Geometry check sheet. Reference: the model listing, model coordinates, mm. A direction names the side the tool comes from. Round coordinates to 2 decimals unless told otherwise and drop trailing zeros. Write each loop counter-clockwise with the first axis right and the second up, starting at its lowest first coordinate (ties: lowest second). Pieces come first, ordered by that corner, then holes. Notation, with made-up numbers: (-40, 88) -> (7, 88) arc R12 ccw to (7, 109) -> close; hole circle Ø10 at (-7.75, 87). An arc over 180 degrees is marked (long way). Return JSON: item names as keys, results as strings. Group by question number.
Autodesk Inventor part; units mm, degrees
ref_plane "YZ Plane" through (0, 0, 0) normal (1, 0, 0) x (0, 1, 0)
ref_plane "XZ Plane" through (0, 0, 0) normal (0, 1, 0) x (-1, 0, 0)
ref_plane "XY Plane" through (0, 0, 0) normal (0, 0, 1) x (1, 0, 0)
sketch "Sketch1" plane through (0, 0, 0) normal (0, 1, 0) x (-1, 0, 0)
  line L0 (-8.3746, 16.5585) -> (42.4254, 16.5585)
  line L1 (42.4254, 16.5585) -> (42.4254, 14.0185)
  line L2 (42.4254, 14.0185) -> (33.5354, 14.0185)
  line L3 (33.5354, 14.0185) -> (33.5354, -11.3815)
  line L4 (33.5354, -11.3815) -> (42.4254, -11.3815)
  line L5 (42.4254, -11.3815) -> (42.4254, -13.9215)
  line L6 (42.4254, -13.9215) -> (-8.3746, -13.9215)
  line L7 (-8.3746, 16.5585) -> (-8.3746, 14.0185)
  line L8 (-8.3746, 14.0185) -> (23.3754, 14.0185)
  line L9 (23.3754, 14.0185) -> (23.3754, -11.3815)
  line L10 (23.3754, -11.3815) -> (-8.3746, -11.3815)
  line L11 (-8.3746, -11.3815) -> (-8.3746, -13.9215)
  point P0 (0, 0)
  dimension "d0" = 30.48
  dimension "d1" = 2.54
  dimension "d2" = 2.54
  dimension "d4" = 2.54
  dimension "d5" = 2.54
  dimension "d6" = 8.89
  dimension "d7" = 50.8
  dimension "d8" = 31.75
extrude "Extrusion1" add sketch "Sketch1" along normal blind 25.4
sketch "Sketch4" plane through (8.3746, 0, -13.9215) normal (0, 0, -1) x (-1, 0, 0)
  line L0 (50.8, 0) -> (0, 0)
  line L1 (50.8, 0) -> (50.8, 25.4)
  line L2 (0, 25.4) -> (50.8, 25.4)
  line L3 (50.8, 25.4) -> (31.75, 25.4)
  line L4 (31.75, 25.4) -> (31.75, 0)
  line L5 (31.75, 0) -> (50.8, 0)
  line L6 (50.8, 0) -> (50.8, 25.4)
  point P0 (8.3746, 0)
  dimension "d56" = 19.05
extrude "Extrusion3" add sketch "Sketch4" along normal blind 13.97
sketch "Sketch5" plane through (-42.4254, 0, 16.5585) normal (0, 0, 1) x (1, 0, 0)
  line L0 (50.8, 0) -> (50.8, 25.4)
  line L1 (50.8, 0) -> (0, 0)
  point P0 (40.64, 12.7)
  dimension "d11" = 10.16
  dimension "d12" = 12.7
hole "Hole1" at (-1.7854, 12.7, 16.5585) direction (0, 0, -1) diameter 9.779 end through all
sketch "Sketch6" plane through (-42.4254, 0, 16.5585) normal (0, 0, 1) x (1, 0, 0)
  line L0 (0, 0) -> (0, 25.4)
  line L1 (50.8, 0) -> (0, 0)
  point P0 (4, 4)
  dimension "d20" = 4
  dimension "d21" = 4
hole "Hole2" at (-38.4254, 4, 16.5585) direction (0, 0, -1) diameter 4.5 end through all
sketch "Sketch2" plane through (-42.4254, 0, 16.5585) normal (0, 0, 1) x (1, 0, 0)
  circle A0 centre (40.64, 12.7) radius 4.8895
  line L0 (40.64, 22.225) -> (40.64, 3.175) construction
  circle A1 centre (40.64, 12.7) radius 4.8895 construction
  line L1 (40.64, 12.7) -> (33.9048, 19.4352) construction
  line L2 (40.64, 12.7) -> (33.9048, 5.9648) construction
  line L3 (40.64, 12.7) -> (47.3752, 5.9648) construction
  line L4 (40.64, 12.7) -> (47.3752, 19.4352) construction
  point P0 (42.4254, 0)
  dimension "d29" = 9.525
  dimension "d30" = 0
  dimension "d33" = 360
  dimension "d60" = 45
  dimension "d63" = 360
hole "Hole3" at (-1.7854, 3.175, 16.5585) at (-1.7854, 22.225, 16.5585) at (-8.5206, 5.9648, 16.5585) at (-8.5206, 19.4352, 16.5585) at (4.9498, 19.4352, 16.5585) at (4.9498, 5.9648, 16.5585) direction (0, 0, -1) diameter 2.794 end through all
fillet "Fillet2" radius 3.175 8 edges at (-42.4254, 0, -19.6365) (-42.4254, 0, 15.2885) (-23.3754, 12.7, 14.0185) (-23.3754, 12.7, -11.3815) (8.3746, 0, -12.6515) (8.3746, 25.4, -12.6515) (8.3746, 25.4, 15.2885) (8.3746, 0, 15.2885)
hole "Hole4" at (-33.5354, 22.1488, 1.9535) direction (1, 0, 0) diameter 3.81 end through all
sketch "Sketch7" plane through (8.3746, 0, -27.8915) normal (0, 0, -1) x (-1, 0, 0)
  circle A0 centre (46.0375, 19.1807) radius 1.45
  circle A1 centre (46.0375, 12.5767) radius 1.524
  line L0 (50.8, 3.175) -> (50.8, 25.4) construction
  line L1 (31.75, 25.4) -> (31.75, 0) construction
  line L2 (50.8, 25.4) -> (31.75, 25.4) construction
  point P0 (8.3746, 0)
  dimension "d65" = 2.9
  dimension "d66" = 3.048
  dimension "d67" = 6.604
  dimension "d69" = 4.7625
  dimension "d71" = 6.2193
extrude "Extrusion4" cut sketch "Sketch7" against normal up to surface (16.51 mm away)
sketch "Sketch9" plane through (8.3746, 0, -27.8915) normal (0, 0, -1) x (-1, 0, 0)
  circle A0 centre (38.1, 12.446) radius 1.45
  line L0 (50.8, 25.4) -> (31.75, 25.4)
  line L1 (50.8, 3.175) -> (50.8, 25.4)
  point P0 (8.3746, 0)
  dimension "d78" = 2.9
  dimension "d79" = 12.954
  dimension "d80" = 12.7
extrude "Extrusion6" cut sketch "Sketch9" against normal blind 12.7
sketch "Sketch10" plane through (0, 25.4, 0) normal (0, 1, 0) x (1, 0, 0)
  line L0 (-42.4254, 11.3815) -> (-42.4254, 27.8915)
  line L1 (-23.3754, 13.9215) -> (-23.3754, 27.8915)
  line L2 (-42.4254, 27.8915) -> (-23.3754, 27.8915)
  line L3 (-23.3754, 27.8915) -> (-23.3754, 26.6215)
  line L4 (-23.3754, 26.6215) -> (-42.4254, 26.6215)
  line L5 (-42.4254, 26.6215) -> (-42.4254, 27.8915)
  point P0 (0, 0)
  dimension "d83" = 1.27
extrude "Extrusion7" cut sketch "Sketch10" against normal through all
equation "\"d2\" = d1"
equation "\"d4\" = d1"
equation "\"d5\" = d1"
properties part number "Odometry_Holder with guard mount" material "Gold"
1) Sectioned sample at A-A on x = -13.5. Enter the section's corners in (y, z), and give its area (3 significant figures).
2) Sectioned sample at C-C on y = 21.5. State how many separate pieces and enclosed holes the cut face has, and give its area (3 significant figures).
3) Mould release check, pull along Y, two halves, no side actions. Record for faces 1 (the face through (-33.535, 13, 1)), 2 (the face through (-24, 25.4, -5)), 3 (the face through (-0.935, 4.284, 15.271)), 4 (the face through (-41.471, 0.905, -19.108)): +Y half, -Y half, draft (parallel to the pull), parting line (faces both ways), or undercut.
4) Material ranges on probe 1 along Z at (x, y) = (-4.5, 3.25); probe 2 along X at (y, z) = (12.7, -12.85); probe 3 along Z at (x, y) = (-37, 15.25), recorded low to high. Write a range as [from, to].
5) Go/stop test with flat-tipped pins: P1, Ø10, axis at y = 18.5, z = -21, coming from the +X side; P2, Ø12.5, axis at x = -10, y = 13.5, coming from the -Z side; P3, Ø10, axis at y = 2.5, z = 7.5, coming from the -X side. Record where each tip stops, or that it passes through.
6) Tool access check on faces 5 (the face through (-36, 13, -11.382)), 6 (the face through (-8, 13, -13.922)), 7 (the face through (8.375, 13, 15)), 8 (the face through (-22.47, 12.878, 13.064)), 9 (the face through (-36.51, 18.3, -19.11)). Record the directions out of +Z, -Z, +X, -X, +Y, -Y that give a thin tool (end or side, any length) a straight path to the whole face; none if there is none.
7) Sectioned sample at B-B on x = -37. Enter the section's corners in (y, z).
Evaluation:
{
 "1": {"outline": "(0, -13.92) -> (25.4, -13.92) -> (25.4, -11.38) -> (0, -11.38) -> close; (0, 14.02) -> (25.4, 14.02) -> (25.4, 16.56) -> (0, 16.56) -> close", "area": "129 mm2"},
 "2": {"separate pieces": "4", "enclosed holes": "0", "area": "714 mm2"},
 "3": {"face 1": "draft", "face 2": "+Y half", "face 3": "undercut", "face 4": "-Y half"},
 "4": {"probe 1": "z = [-13.92, -11.38], [14.02, 16.56]", "probe 2": "x = [-42.43, -39.18], [-36.14, -6.67], [3.1, 8.37]", "probe 3": "z = [-26.62, -11.38], [14.02, 16.56]"},
 "5": {"P1": "stops at x = -23.38", "P2": "stops at z = -13.92", "P3": "stops at x = -33.54"},
 "6": {"face 5": "-X, +Y, -Y", "face 6": "-Z, +X, +Y, -Y", "face 7": "+Z, -Z, +X, +Y, -Y", "face 8": "+X, +Y, -Y", "face 9": "-Z"},
 "7": {"outline": "(0, -26.62) -> (2.26, -26.62) -> (2.26, -11.38) -> (0, -11.38) -> close; (0, 14.02) -> (2.26, 14.02) -> (2.26, 16.56) -> (0, 16.56) -> close; (5.74, -26.62) -> (11.2, -26.62) -> (11.2, -11.38) -> (5.74, -11.38) -> close; (5.74, 14.02) -> (25.4, 14.02) -> (25.4, 16.56) -> (5.74, 16.56) -> close; (13.95, -26.62) -> (17.89, -26.62) -> (17.89, -11.38) -> (13.95, -11.38) -> close; (20.47, -26.62) -> (25.4, -26.62) -> (25.4, -11.38) -> (20.47, -11.38) -> close"}
}
